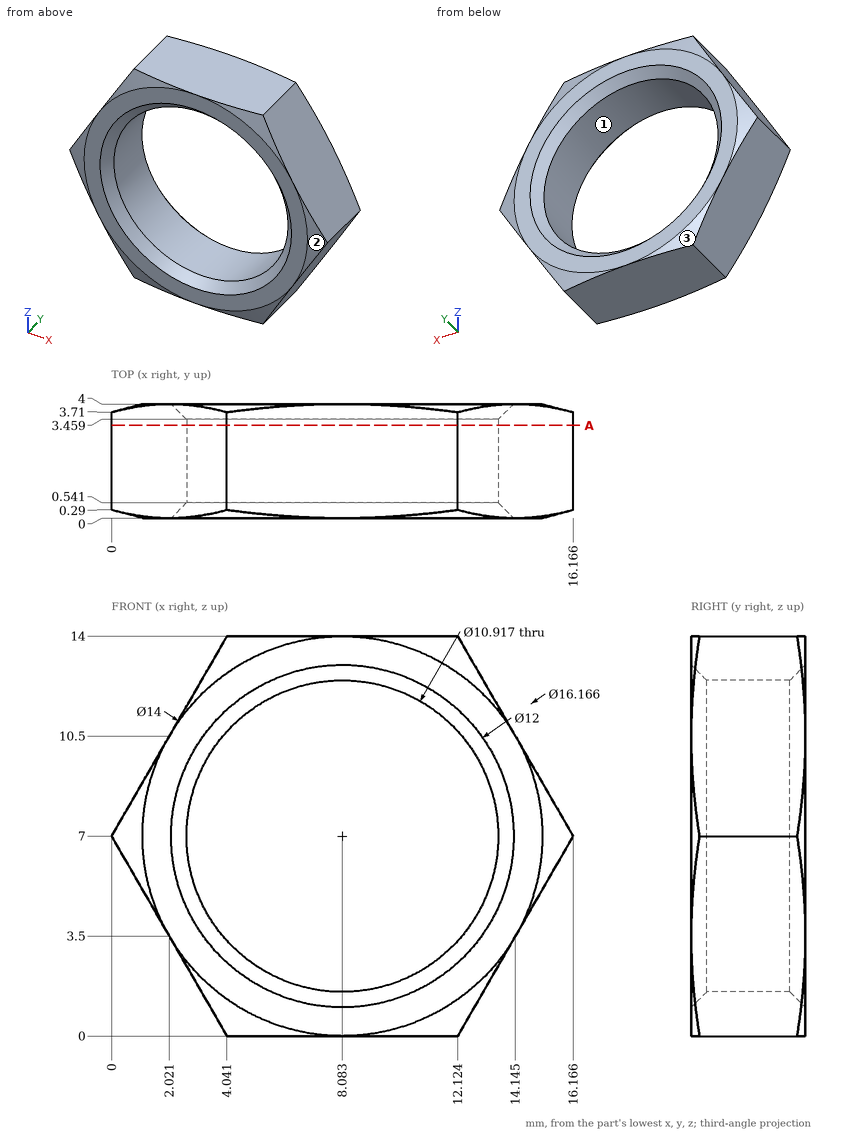
The drawing under review shows one solid part. Ordinate dimensions are in mm from its lowest x, y, z. Give positions to 0.01 mm unless a question says otherwise; leave off trailing zeros. Loops run counter-clockwise (first coordinate to the right, second up) from the corner with the lowest first, then second, coordinate; pieces in that order, holes last. Notation, with made-up numbers: M -36.75,76.5 L 5.25,76.5 A17 cw 5.25,102.5 Z; hole C 64,52.5 d2. An arc over 180 degrees is marked long. Return JSON: item names as keys, results as strings. Group by question number.
Item 1: Insertion check: pin 1 Ø1.5 at (y, z) = (1.5, 9) entering from +X (1 decimal); pin 2 Ø2 at (x, z) = (10.5, 1.5) entering from -Y; pin 3 Ø6.5 at (x, z) = (8.08, 7) entering from +Y; pin 4 Ø1 at (y, z) = (0.5, 9.5) entering from +X. Each pin has a flat end and moves straight along its axis. Give the tip position at first contact, or say it passes through.
Item 2: For probe 1 along X at (y, z) = (0.4, 9.5) (1 decimal); probe 2 along X at (y, z) = (0.25, 6) (1 decimal); probe 3 along Z at (x, y) = (12, 3), list the stretches that pass through material, from the lowest coordinate up.
Item 3: We need section A-A (y = 3.25). Give the boundary of the cut face in (x, z) (1 decimal).
Item 4: Mouldability with a two-part tool opening along Z and no side actions: class the marked faces 1, 2 and 3 as released by +Z, released by -Z, zero draft, split by the parting line, or undercut.
Output:
{
 "1": {"pin 1": "stops at x = 15.4", "pin 2": "stops at y = 0", "pin 3": "passes through", "pin 4": "stops at x = 15.01"},
 "2": {"probe 1": "x = 1.4 to 3.1, 13.1 to 14.7", "probe 2": "x = 0.6 to 2.4, 13.7 to 15.6", "probe 3": "z = 0 to 3.2, 10.8 to 14"},
 "3": {"outline": "M 0,7 L 4,0 L 12.1,0 L 16.2,7 L 12.1,14 L 4,14 Z; hole C 8.1,7 d10.9"},
 "4": {"face 1": "undercut", "face 2": "split by the parting line", "face 3": "released by -Z"}
}
